For this review, take the finished solid that the model builds, in its own axes (mm). Face numbers are marked on the shaded views. Coordinates: 2 decimals unless noted, no trailing zeros. Order: outer loops, then holes, each group sorted by start corner. A loop starts at its lowest first (then second) coordinate and runs counter-clockwise, first axis right, second up. Notation, with made-up numbers: (63, 61.5) -> (93, 61.5) arc R38 cw to (93, 100.5) -> close; hole circle Ø7 at (78.5, 12). An arc over 180 degrees is marked (long way). Return JSON: item names as keys, results as strings. Group by question number.
Item 1: Take a section at B-B (z = 0). Write out the cut boundary in (x, y), then the cut area to 3 significant figures.
Item 2: Draft analysis for pull direction Z (two halves, no side actions). For the marked faces 1, 2 and 3, state which applies: +Z half, -Z half, draft (parallel to the pull), parting line (faces both ways), or undercut.
Item 3: Insertion check: pin 1 (2 mm diameter, centred on x = 27.5, z = -35.5, fed in from +Y); pin 2 (3 mm diameter, centred on y = 7.5, z = -23, fed in from +X); pin 3 (1 mm diameter, centred on y = 14.5, z = -30, fed in from -X); pin 4 (4 mm diameter, centred on x = -2, z = -3.5, fed in from -Y). Each pin has a flat end and moves straight along its axis. Give the tip position at first contact, or say it passes through.
Item 4: Take a section at C-C (y = 15). Write out the cut boundary in (x, z), then the cut area to 3 significant figures.
Item 5: For line 1 along X through (y, z) = (14.5, 0); line 2 along Y through (x, z) = (10.5, -18); line 3 along Z through (x, y) = (3, 11.5), list the stretches that pass through material, from the lowest coordinate up.
Item 6: Take a section at D-D (x = 13). Write out the cut boundary in (y, z).
Item 7: Take a section at A-A (x = 0). Write out the cut boundary in (y, z), then the cut area to 3 significant figures.
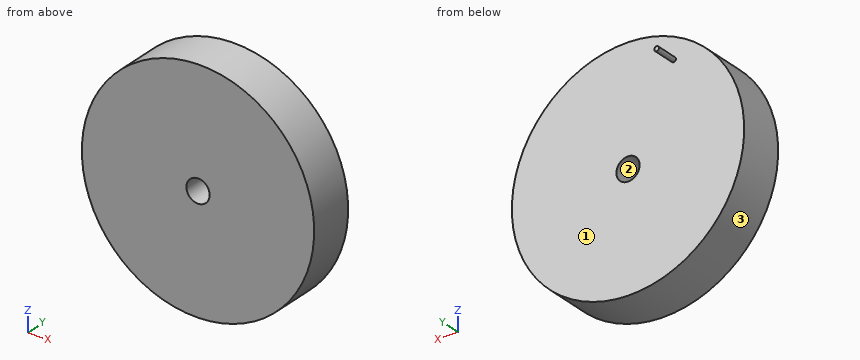
```python
from build123d import *

# Parameters (mm, degrees)
SKETCH1_R           = 50
BOSS_EXTRUDE1_DEPTH = 20
SKETCH4_R           = 5
CUT_EXTRUDE2_DEPTH  = 20
SKETCH5_R           = 1
BOSS_EXTRUDE2_DEPTH = 10


with BuildPart() as part:
    # Sketch1 → Boss-Extrude1 (new body)
    with BuildSketch(Plane(origin=(0, 0, 0), x_dir=(1, 0, 0), z_dir=(0, 1, 0))):
        with Locations(Location((0, 0, 0), (0, 0, 270))):
            Circle(SKETCH1_R)
    extrude(amount=BOSS_EXTRUDE1_DEPTH)

    # Sketch4 → Cut-Extrude2 (cut)
    with BuildSketch(Plane.XZ):
        with Locations(Location((0, 0, 0), (0, 0, 270))):
            Circle(SKETCH4_R)
    extrude(amount=-CUT_EXTRUDE2_DEPTH, mode=Mode.SUBTRACT)

    # Sketch5 → Boss-Extrude2 (add)
    with BuildSketch(Plane(origin=(0, 20, 0), x_dir=(1, 0, 0), z_dir=(0, 1, 0))):
        with Locations(Location((-19.611481927, -36.877253926, 0), (0, 0, 270))):
            Circle(SKETCH5_R)
    extrude(amount=BOSS_EXTRUDE2_DEPTH)


solid = part.part
```
Findings below:
{
 "1": {"outline": "(-50, 0) -> (-5, 0) -> (-5, 20) -> (-50, 20) -> close; (5, 0) -> (50, 0) -> (50, 20) -> (5, 20) -> close", "area": "1,800 mm2"},
 "2": {"face 1": "draft", "face 2": "undercut", "face 3": "parting line"},
 "3": {"pin 1": "stops at y = 20", "pin 2": "stops at x = 45.14", "pin 3": "stops at x = -40.37", "pin 4": "stops at y = 0"},
 "4": {"outline": "circle Ø100 at (0, 0); hole circle Ø10 at (0, 0)", "area": "7,780 mm2"},
 "5": {"line 1": "x = -50 to -5, 5 to 50", "line 2": "y = 0 to 20", "line 3": "z = -49.91 to -4, 4 to 49.91"},
 "6": {"outline": "(0, -48.28) -> (20, -48.28) -> (20, 48.28) -> (0, 48.28) -> close"},
 "7": {"outline": "(0, -50) -> (20, -50) -> (20, -5) -> (0, -5) -> close; (0, 5) -> (20, 5) -> (20, 50) -> (0, 50) -> close", "area": "1,800 mm2"}
}
